Work out the finished part from the listing and answer in its coordinate system (mm). A direction names the side the tool comes from. Coordinates: 2 decimals unless noted, no trailing zeros. Loops run counter-clockwise (first coordinate to the right, second up) from the corner with the lowest first, then second, coordinate; pieces in that order, holes last. Notation, with made-up numbers: (41.5, 60) -> (89.5, 60) arc R17 cw to (89.5, 86) -> close; hole circle Ø8 at (-17.5, 63.5). An arc over 180 degrees is marked (long way). Use a Markdown table: item, result. Add a question column.
```python
from build123d import *

# Parameters (mm, degrees)
AUFSATZ_LINEAR_AUSTRAGEN1_DEPTH = 10
SKIZZE2_W                       = 25
SKIZZE2_H                       = 40
AUFSATZ_LINEAR_AUSTRAGEN2_DEPTH = 100
SKIZZE3_R                       = 7.5
SCHNITT_LINEAR_AUSTRAGEN1_DEPTH = 285.604989415
SKIZZE4_W                       = 25
SKIZZE4_H                       = 200
AUFSATZ_LINEAR_AUSTRAGEN3_DEPTH = 200
SCHNITT_LINEAR_AUSTRAGEN4_REACH = 365.992
SCHNITT_LINEAR_AUSTRAGEN3_DEPTH = 364.992344743
SCHNITT_LINEAR_AUSTRAGEN5_DEPTH = 6
SKIZZE9_R                       = 30
AUFSATZ_LINEAR_AUSTRAGEN4_DEPTH = 20


with BuildPart() as part:
    # Skizze1 → Aufsatz-Linear austragen1 (new body)
    with BuildSketch(Plane(origin=(0, 0, 0), x_dir=(1, 0, 0), z_dir=(0, 1, 0))):
        Polygon((0, 0), (240, 0), (240, 200), (185, 200), (185, 50), (55, 50), (55, 200), (0, 200), align=None)
    extrude(amount=AUFSATZ_LINEAR_AUSTRAGEN1_DEPTH)

    # Skizze2 → Aufsatz-Linear austragen2 (add)
    with BuildSketch(Plane(origin=(0, 10, 0), x_dir=(1, 0, 0), z_dir=(0, 1, 0))):
        with Locations((157.5, 20)):
            Rectangle(SKIZZE2_W, SKIZZE2_H)
        with Locations((82.5, 20)):
            Rectangle(SKIZZE2_W, SKIZZE2_H)
    extrude(amount=AUFSATZ_LINEAR_AUSTRAGEN2_DEPTH)

    # Skizze3 → Schnitt-Linear austragen1 (cut, through all)
    with BuildSketch(Plane(origin=(170, 0, 0), x_dir=(0, 0, -1), z_dir=(1, 0, 0))):
        with Locations((20, 110)):
            Circle(SKIZZE3_R)
    extrude(amount=-SCHNITT_LINEAR_AUSTRAGEN1_DEPTH, mode=Mode.SUBTRACT)

    # Skizze4 → Aufsatz-Linear austragen3 (add)
    with BuildSketch(Plane(origin=(0, 10, 0), x_dir=(1, 0, 0), z_dir=(0, 1, 0))):
        with Locations((207.478242177, 100)):
            Rectangle(SKIZZE4_W, SKIZZE4_H)
        with Locations((32.521757823, 100)):
            Rectangle(SKIZZE4_W, SKIZZE4_H)
    extrude(amount=AUFSATZ_LINEAR_AUSTRAGEN3_DEPTH)

    # Skizze7 → Schnitt-Linear austragen4 (cut, up to next)
    with BuildSketch(Plane(origin=(219.978242177, 0, 0), x_dir=(0, 0, -1), z_dir=(1, 0, 0)), mode=Mode.PRIVATE) as schnitt_linear_austragen4_sk1:
        Polygon((0, 44.069377938), (136.337930206, 175.975272551), (200, 175.975272551), (200, 225.622509637), (-41.808038164, 225.622509637), align=None)
    schnitt_linear_austragen4_tool1 = extrude(schnitt_linear_austragen4_sk1.sketch, amount=-SCHNITT_LINEAR_AUSTRAGEN4_REACH, mode=Mode.PRIVATE) & part.part
    schnitt_linear_austragen4 = schnitt_linear_austragen4_tool1.solids().sort_by_distance((219.978242, 167.605519, -59.370877))[0]
    add(schnitt_linear_austragen4, mode=Mode.SUBTRACT)

    # Skizze6 → Schnitt-Linear austragen3 (cut, through all)
    with BuildSketch(Plane(origin=(219.978242177, 0, 0), x_dir=(0, 0, -1), z_dir=(1, 0, 0))):
        with BuildLine():
            ThreePointArc((152.985895116, 28.803269607), (174.718481208, 91.551452657), (168.349561926, 157.650443887))
            ThreePointArc((168.349561926, 157.650443887), (161.035471277, 161.408211518), (157.277703645, 154.094120869))
            ThreePointArc((157.277703645, 154.094120869), (163.171287707, 92.928333715), (143.060682227, 34.863271943))
            ThreePointArc((143.060682227, 34.863271943), (144.993287504, 26.870664331), (152.985895116, 28.803269607))
        make_face()
    extrude(amount=-SCHNITT_LINEAR_AUSTRAGEN3_DEPTH, mode=Mode.SUBTRACT)

    # Skizze8 → Schnitt-Linear austragen5 (cut)
    with BuildSketch(Plane(origin=(219.978242177, 0, 0), x_dir=(0, 0, -1), z_dir=(1, 0, 0))):
        with BuildLine():
            ThreePointArc((161.538964629, 23.581052028), (184.669295342, 90.364923006), (177.890755105, 160.715111448))
            ThreePointArc((177.890755105, 160.715111448), (157.970803716, 170.949404697), (147.736510466, 151.029453308))
            ThreePointArc((147.736510466, 151.029453308), (153.220473573, 94.114863367), (134.507612714, 40.085489522))
            ThreePointArc((134.507612714, 40.085489522), (139.771069924, 18.317594818), (161.538964629, 23.581052028))
        make_face()
    schnitt_linear_austragen5 = extrude(amount=-SCHNITT_LINEAR_AUSTRAGEN5_DEPTH, mode=Mode.SUBTRACT)

    # Spiegeln1: Schnitt-Linear austragen4, Schnitt-Linear austragen5 across plane
    add(schnitt_linear_austragen4.mirror(Plane(origin=(120, 0, 0), x_dir=(0, 0, 1), z_dir=(1, 0, 0))), mode=Mode.SUBTRACT)
    add(schnitt_linear_austragen5.mirror(Plane(origin=(120, 0, 0), x_dir=(0, 0, 1), z_dir=(1, 0, 0))), mode=Mode.SUBTRACT)

    # Skizze9 → Aufsatz-Linear austragen4 (add)
    with BuildSketch(Plane.XZ):
        with Locations(Location((120, -31.686005805, 0), (0, 0, 322.37676034))):
            Circle(SKIZZE9_R)
    extrude(amount=AUFSATZ_LINEAR_AUSTRAGEN4_DEPTH)


solid = part.part
```
Item 1: Find the intervals of material crossed by probe 1 along X at (y, z) = (65, -37.5); probe 2 along X at (y, z) = (151.5, -135.5); probe 3 along X at (y, z) = (84, -37.5), in increasing order.
Item 2: Section C-C (z = -108) is taken. Determine the outline of the cut face in (x, y).
Item 3: For a pull along Y with two mould halves and no side action, classify faces 5 (the face through (213, 87, -200)), 6 (the face through (230, 10, -101)), 7 (the face through (22.98, 18.5, -139.48)) as +Y half, -Y half, draft (parallel to the pull), parting line (faces both ways), or undercut.
Item 4: Section D-D (y = 124.5) is taken. Determine the outline of the cut face in (x, z), then the cut area to 3 significant figures.
Item 5: For faces 1 (the face through (157, 59, -40)), 2 (the face through (217.02, 94.916, -153.314)), 3 (the face through (35.655, 90.622, -174.605)), 4 (the face through (194.978, 73, -121)), determine the directions among +Z, -Z, +X, -X, +Y, -Y from which every point of the face is accessible in a straight line to the end or side of a thin tool.
Item 6: Section A-A (y = 98.5) is taken. Count the separate pieces of the cut face and the enclosed holes in it, then the cut area to 3 significant figures.
Item 7: Given pin 1 (4 mm diameter, centred on x = 158.5, z = -33.5, fed in from +Y); pin 2 (13 mm diameter, centred on x = 118.5, z = -57, fed in from +Y); pin 3 (12 mm diameter, centred on y = 81.5, z = -141, fed in from -X); pin 4 (8 mm diameter, centred on x = 80.5, z = -56, fed in from -Y), each flat-ended and moving along its own axis, determine where each tip first touches the part or whether it passes through.
Item 8: Section B-B (x = 120) is taken. Determine the outline of the cut face in (y, z).
Output:
| question | item | result |
|---|---|---|
| 1 | probe 1 | x = 20.02 to 45.02, 70 to 95, 145 to 170, 194.98 to 219.98 |
| 1 | probe 2 | x = 20.02 to 45.02, 194.98 to 219.98 |
| 1 | probe 3 | x = 70 to 95, 145 to 170 |
| 2 | outline | (0, 0) -> (55, 0) -> (55, 10) -> (45.02, 10) -> (45.02, 148.56) -> (20.02, 148.56) -> (20.02, 10) -> (0, 10) -> close; (185, 0) -> (240, 0) -> (240, 10) -> (219.98, 10) -> (219.98, 148.56) -> (194.98, 148.56) -> (194.98, 10) -> (185, 10) -> close |
| 3 | face 5 | draft |
| 3 | face 6 | +Y half |
| 3 | face 7 | undercut |
| 4 | outline | (20.02, -200) -> (45.02, -200) -> (45.02, -175.14) -> (26.02, -175.14) -> (26.02, -185.2) -> (20.02, -185.2) -> close; (20.02, -153.38) -> (26.02, -153.38) -> (26.02, -163.45) -> (45.02, -163.45) -> (45.02, -83.13) -> (20.02, -83.13) -> close; (194.98, -200) -> (219.98, -200) -> (219.98, -185.2) -> (213.98, -185.2) -> (213.98, -175.14) -> (194.98, -175.14) -> close; (194.98, -163.45) -> (213.98, -163.45) -> (213.98, -153.38) -> (219.98, -153.38) -> (219.98, -83.13) -> (194.98, -83.13) -> close |
| 4 | area | 5,020 mm2 |
| 5 | face 1 | -Z, +Y |
| 5 | face 2 | +X |
| 5 | face 3 | +X, -X |
| 5 | face 4 | +Z, -Z, +Y |
| 6 | separate pieces | 6 |
| 6 | enclosed holes | 0 |
| 6 | area | 8,360 mm2 |
| 7 | pin 1 | stops at y = 110 |
| 7 | pin 2 | stops at y = 0 |
| 7 | pin 3 | stops at x = 20.02 |
| 7 | pin 4 | passes through |
| 8 | outline | (-20, -61.69) -> (0, -61.69) -> (0, -50) -> (10, -50) -> (10, 0) -> (0, 0) -> (0, -1.69) -> (-20, -1.69) -> close |
